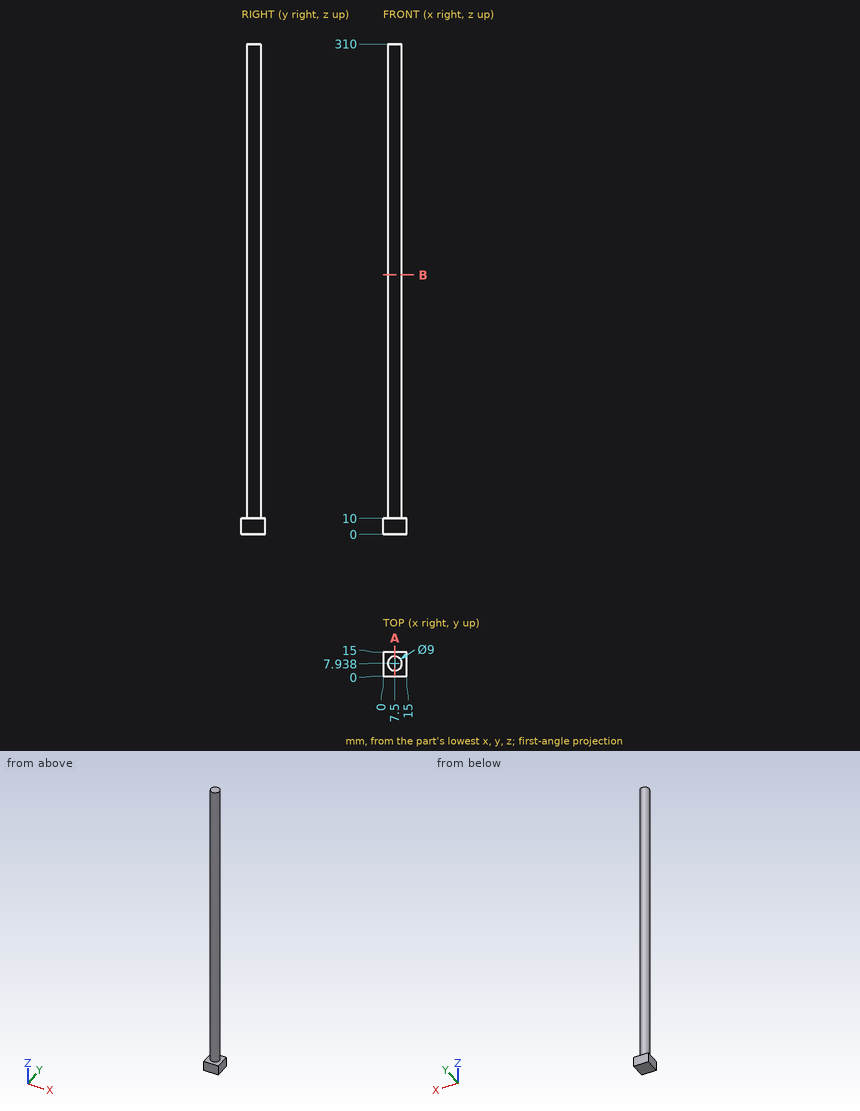
For this review, use the dimensioned drawing (mm, ordinates from the lowest corner) and the shaded views. Give positions to 0.01 mm unless a question says otherwise; leave off trailing zeros. Order: outer loops, then holes, each group sorted by start corner. A loop starts at its lowest first (then second) coordinate and runs counter-clockwise, first axis right, second up. Notation, with made-up numbers: (87.5, 19) - (143.5, 19) arc R27 cw to (143.5, 40) - close; hole circle Ø6 at (-24.75, 77). An arc over 180 degrees is marked (long way). Use CSV: the item, a comma, the result in double quotes. Start each with the question number.
Q1. For P1, Ø8, axis at y = 7.5, z = 267, coming from the -X side; P2, Ø8, axis at x = 5, z = 32, coming from the -Y side; P3, Ø2, axis at x = 6.5, z = 126.5, coming from the +Y side, all flat-tipped, find the tip position at first contact; note any pin that passes through.
Q2. Take a section at A-A (x = 7.5). State the section outline as (y, z) points.
Q3. Take a section at B-B (z = 164). State the section outline as (x, y) points, and give its area (3 significant figures).
Q4. For line 1 (Y direction, x = 8.25, z = 213.5) (1 decimal); line 2 (Z direction, x = 1.25, y = 1.75); line 3 (X direction, y = 12, z = 70.5) (1 decimal), list the stretches that pass through material, from the lowest coordinate up.
Calculated:
1,P1,"stops at x = 3"
1,P2,"stops at y = 3.44"
1,P3,"stops at y = 12.44"
2,outline,"(0, 0) - (15, 0) - (15, 10) - (12.44, 10) - (12.44, 310) - (3.44, 310) - (3.44, 10) - (0, 10) - close"
3,outline,"circle Ø9 at (7.5, 7.94)"
3,area,"63.6 mm²"
4,line 1,"y = 3.5 to 12.4"
4,line 2,"z = 0 to 10"
4,line 3,"x = 5.6 to 9.4"
